Check sheet for the modelled part. Datum: model origin and axes. Units: mm. A direction names the side the tool comes from. Round coordinates to 2 decimals unless told otherwise and drop trailing zeros. Order: outer loops, then holes, each group sorted by start corner. A loop starts at its lowest first (then second) coordinate and runs counter-clockwise, first axis right, second up.
(1) Mould release check, pull along Y, two halves, no side actions. Record for faces 5 (the flat face through (-399, -56.483, 400)), 6 (the flat face through (838.2, -210, 42)): released by +Y, released by -Y, zero draft, split by the parting line, or undercut.
(2) Sectioned sample at D-D, the plane z = -162.5. Enter the section's corners in (x, y), and give its area (3 significant figures).
(3) Sectioned sample at C-C, the plane z = 423. Enter the section's corners in (x, y).
(4) Sectioned sample at B-B, the plane x = 544. Enter the section's corners in (y, z).
(5) Tool access check on faces 1 (the flat face through (-724.921, -442, 398)), 2 (the flat face through (661.919, -442, -17)), 3 (the flat face through (-57, -442, -317.474)), 4 (the flat face through (235.199, -442, -17)). Record the directions out of +Z, -Z, +X, -X, +Y, -Y that give a thin tool (end or side, any length) a straight path to the whole face; none if there is none.
(6) Thickness scan on probe 1 along X at (y, z) = (-447.5, -301.5); probe 2 along X at (y, z) = (-248, 458); probe 3 along Z at (x, y) = (357, -439.5). Record the ranges inside material, lowest first.
(7) Sectioned sample at A-A, the plane y = -145.5. Enter the section's corners in (x, z), and give its area (3 significant figures).
(8) Depth check by flat-ended pin: pin 1 (15 mm diameter, centred on x = 362, y = -436, fed in from +Z); pin 2 (5 mm diameter, centred on x = 168.5, z = 100, fed in from -Y); pin 3 (12 mm diameter, centred on x = -328, y = -464.5, fed in from +Z). Enter the tip coordinate at first touch or a pass-through.
```python
from build123d import *

# Parameters (mm, degrees)
F0_W     = 1676.4
F0_H     = 914.4
F1_DEPTH = 426.72
F2_W     = 426.72
F2_H     = 609.6
F2_H_2   = 152.4
F3_DEPTH = 30.48
F4_W     = 15.24
F4_H     = 121.92
F5_DEPTH = 45.72
F6_W     = 457.2
F6_H     = 304.8
F7_DEPTH = 213.36


with BuildPart() as f1:
    # F0 (on Front) → F1 (new body)
    with BuildSketch(Plane.XZ):
        with Locations((2e-06, 48.286399)):
            Rectangle(F0_W, F0_H)
    extrude(amount=F1_DEPTH)

    # F2 (on face) → F3 (join)
    with BuildSketch(Plane.XZ.offset(426.72)):
        with Locations((-511.561048, -12.673601)):
            Rectangle(F2_W, F2_H)
        with Locations((-54.361048, -12.673601)):
            Rectangle(F2_W, F2_H)
        with Locations((448.558952, -12.673601)):
            Rectangle(F2_W, F2_H)
        with Locations((-511.561048, 398.806399)):
            Rectangle(F2_W, F2_H_2)
        with Locations((-54.361048, 398.806399)):
            Rectangle(F2_W, F2_H_2)
        with Locations((448.558952, 398.806399)):
            Rectangle(F2_W, F2_H_2)
    extrude(amount=F3_DEPTH)

    # F4 (on face) → F5 (join)
    with BuildSketch(Plane.XZ.offset(426.72)):
        with Locations((-327.157048, 60.96)):
            Rectangle(F4_W, F4_H)
        with Locations((-238.765048, 60.96)):
            Rectangle(F4_W, F4_H)
        with Locations((632.962952, 61.087999)):
            Rectangle(F4_W, F4_H)
    extrude(amount=F5_DEPTH)

    # F6 (on face) → F7 (cut)
    with BuildSketch(Plane.XY.offset(505.486399)):
        with Locations((-396.239998, -208.883211)):
            Rectangle(F6_W, F6_H)
    extrude(amount=-F7_DEPTH, mode=Mode.SUBTRACT)


solid = f1.part
```
Derived:
1. face 5: undercut
1. face 6: zero draft
2. outline: (-838.2, -426.72) - (-724.92, -426.72) - (-724.92, -457.2) - (-298.2, -457.2) - (-298.2, -426.72) - (-267.72, -426.72) - (-267.72, -457.2) - (159, -457.2) - (159, -426.72) - (235.2, -426.72) - (235.2, -457.2) - (661.92, -457.2) - (661.92, -426.72) - (838.2, -426.72) - (838.2, 0) - (-838.2, 0) - close
2. area: 754,000 mm2
3. outline: (-838.2, -426.72) - (-724.92, -426.72) - (-724.92, -457.2) - (-298.2, -457.2) - (-298.2, -426.72) - (-267.72, -426.72) - (-267.72, -457.2) - (159, -457.2) - (159, -426.72) - (235.2, -426.72) - (235.2, -457.2) - (661.92, -457.2) - (661.92, -426.72) - (838.2, -426.72) - (838.2, 0) - (-838.2, 0) - close; hole (-624.84, -361.28) - (-167.64, -361.28) - (-167.64, -56.48) - (-624.84, -56.48) - close
4. outline: (-457.2, -317.47) - (-426.72, -317.47) - (-426.72, -408.91) - (0, -408.91) - (0, 505.49) - (-426.72, 505.49) - (-426.72, 475.01) - (-457.2, 475.01) - (-457.2, 322.61) - (-426.72, 322.61) - (-426.72, 292.13) - (-457.2, 292.13) - close
5. face 1: +Z, -Z, -X, -Y
5. face 2: +Z, -Z, +X, -Y
5. face 3: -Z, +X, -X, -Y
5. face 4: +Z, -Z, -Y
6. probe 1: x = -724.92 to -298.2, -267.72 to 159, 235.2 to 661.92
6. probe 2: x = -838.2 to -624.84, -167.64 to 838.2
6. probe 3: z = -317.47 to 292.13, 322.61 to 475.01
7. outline: (-838.2, -408.91) - (838.2, -408.91) - (838.2, 505.49) - (-167.64, 505.49) - (-167.64, 292.13) - (-624.84, 292.13) - (-624.84, 505.49) - (-838.2, 505.49) - close
7. area: 1,440,000 mm2
8. pin 1: stops at z = 475.01
8. pin 2: stops at y = -426.72
8. pin 3: stops at z = 121.92
